Can you work these out from the model? Positions are in its coordinate system, mm. Give positions to 0.01 mm unless a question says otherwise; leave off trailing zeros. Order: outer loops, then holes, each group sorted by start corner. A loop starts at its lowest first (then second) coordinate and runs counter-clockwise, first axis right, second up. Notation, with made-up numbers: (43, 76) -> (64, 76) arc R36 cw to (64, 113) -> close; hole circle Ø2 at (67.5, 81). An arc over 180 degrees is marked (long way). Answer as a JSON object with one key per item and string values.
```python
from build123d import *

# Parameters (mm, degrees)
BOSS_EXTRUDE1_DEPTH                          = 2.5
CSK_FOR_M3_COUNTERSUNK_FLAT_HEAD_SCR_2_COUNT = 2
CSK_FOR_M3_COUNTERSUNK_FLAT_HEAD_SCR_2_PITCH = 33.1
CSK_FOR_M3_COUNTERSUNK_FLAT_HEAD_SCR_3_COUNT = 2
CSK_FOR_M3_COUNTERSUNK_FLAT_HEAD_SCR_3_PITCH = 73.026544956
CSK_FOR_M3_COUNTERSUNK_FLAT_HEAD_SCR_4_COUNT = 2
CSK_FOR_M3_COUNTERSUNK_FLAT_HEAD_SCR_4_PITCH = 146.05
CSK_FOR_M3_COUNTERSUNK_FLAT_HEAD_SCR_5_COUNT = 2
CSK_FOR_M3_COUNTERSUNK_FLAT_HEAD_SCR_5_PITCH = 149.753839684
CUT_EXTRUDE1_DEPTH                           = 86.383473485


with BuildPart() as part:
    # Sketch2 → Boss-Extrude1 (new body)
    with BuildSketch(Plane.XY):
        with BuildLine():
            Line((-75.2, -11.559818622), (75.2, -11.559818622))
            ThreePointArc((75.2, -11.559818622), (75.907106781, -11.266925403), (76.2, -10.559818622))
            Line((76.2, -10.559818622), (76.2, 37.440181378))
            ThreePointArc((76.2, 37.440181378), (75.907106781, 38.147288159), (75.2, 38.440181378))
            Line((75.2, 38.440181378), (-75.2, 38.440181378))
            ThreePointArc((-75.2, 38.440181378), (-75.907106781, 38.147288159), (-76.2, 37.440181378))
            Line((-76.2, 37.440181378), (-76.2, -10.559818622))
            ThreePointArc((-76.2, -10.559818622), (-75.907106781, -11.266925403), (-75.2, -11.559818622))
        make_face()
    extrude(amount=BOSS_EXTRUDE1_DEPTH)

    # Sketch5 → CSK for M3 Countersunk Flat Head Screw1 (revolve, cut)
    with BuildSketch(Plane(origin=(-73.025, 33.440181378, 2.5), x_dir=(0, -1, 0), z_dir=(1, 0, 0))):
        Polygon((0, 0), (0, 2.5), (1.7, 2.5), (1.7, 1.45), (3.15, 0), align=None)
    csk_for_m3_countersunk_flat_head_screw1 = revolve(axis=Axis((-73.025, 33.440181378, 8.85), (0, 0, -1)), mode=Mode.SUBTRACT)

    # CSK for M3 Countersunk Flat Head Scr 2: CSK for M3 Countersunk Flat Head Screw1 ×2
    with Locations(*[(0, -i * CSK_FOR_M3_COUNTERSUNK_FLAT_HEAD_SCR_2_PITCH, 0) for i in range(1, CSK_FOR_M3_COUNTERSUNK_FLAT_HEAD_SCR_2_COUNT)]):
        add(csk_for_m3_countersunk_flat_head_screw1, mode=Mode.SUBTRACT)

    # CSK for M3 Countersunk Flat Head Scr 3: CSK for M3 Countersunk Flat Head Screw1 ×2
    with Locations(*[Vector(0.9999788439186126, 0.006504745590340633, 0) * (i * CSK_FOR_M3_COUNTERSUNK_FLAT_HEAD_SCR_3_PITCH) for i in range(1, CSK_FOR_M3_COUNTERSUNK_FLAT_HEAD_SCR_3_COUNT)]):
        add(csk_for_m3_countersunk_flat_head_screw1, mode=Mode.SUBTRACT)

    # CSK for M3 Countersunk Flat Head Scr 4: CSK for M3 Countersunk Flat Head Screw1 ×2
    with Locations(*[(i * CSK_FOR_M3_COUNTERSUNK_FLAT_HEAD_SCR_4_PITCH, 0, 0) for i in range(1, CSK_FOR_M3_COUNTERSUNK_FLAT_HEAD_SCR_4_COUNT)]):
        add(csk_for_m3_countersunk_flat_head_screw1, mode=Mode.SUBTRACT)

    # CSK for M3 Countersunk Flat Head Scr 5: CSK for M3 Countersunk Flat Head Screw1 ×2
    with Locations(*[Vector(0.9752671471296755, -0.22102939109888511, 0) * (i * CSK_FOR_M3_COUNTERSUNK_FLAT_HEAD_SCR_5_PITCH) for i in range(1, CSK_FOR_M3_COUNTERSUNK_FLAT_HEAD_SCR_5_COUNT)]):
        add(csk_for_m3_countersunk_flat_head_screw1, mode=Mode.SUBTRACT)

    # Sketch6 → Cut-Extrude1 (cut, through all)
    with BuildSketch(Plane.XY.offset(2.5)):
        with BuildLine():
            ThreePointArc((-12.7, 7.935569815), (-16, 20.035569815), (-19.3, 7.935569815))
            Line((-19.3, 7.935569815), (-12.7, 7.935569815))
        make_face()
        with BuildLine():
            ThreePointArc((19.3, 7.935569815), (16, 20.035569815), (12.7, 7.935569815))
            Line((12.7, 7.935569815), (19.3, 7.935569815))
        make_face()
    extrude(amount=-CUT_EXTRUDE1_DEPTH, mode=Mode.SUBTRACT)


solid = part.part
```
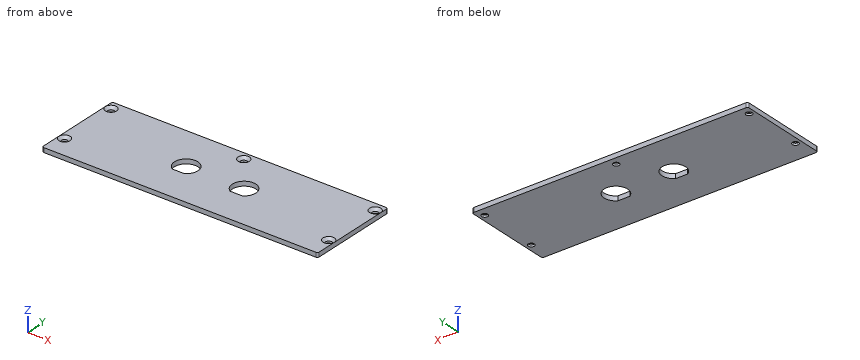
1. If we section it at D-D on x = 16: Please give me the cut outline in (y, z).
Worked answers:
{"outline": "(-11.56, 0) -> (7.94, 0) -> (7.94, 2.5) -> (-11.56, 2.5) -> close; (20.04, 0) -> (38.44, 0) -> (38.44, 2.5) -> (20.04, 2.5) -> close"}
2. If we section it at B-B on y = 13.5: Please give me the cut outline in (x, z).
Worked answers:
{"outline": "(-76.2, 0) -> (-22.5, 0) -> (-22.5, 2.5) -> (-76.2, 2.5) -> close; (-9.5, 0) -> (9.5, 0) -> (9.5, 2.5) -> (-9.5, 2.5) -> close; (22.5, 0) -> (76.2, 0) -> (76.2, 2.5) -> (22.5, 2.5) -> close"}
3. If we section it at C-C on z = 1.8: Please give me the cut outline in (x, y) (3 decimals).
Worked answers:
{"outline": "(-76.2, -10.56) arc R1 ccw to (-75.2, -11.56) -> (75.2, -11.56) arc R1 ccw to (76.2, -10.56) -> (76.2, 37.44) arc R1 ccw to (75.2, 38.44) -> (-75.2, 38.44) arc R1 ccw to (-76.2, 37.44) -> close; hole circle Ø4.9 at (-73.025, 0.34); hole circle Ø4.9 at (-73.025, 33.44); hole (-19.3, 7.936) -> (-12.7, 7.936) arc R6.5 ccw (long way) to start; hole circle Ø4.9 at (0, 33.915); hole (12.7, 7.936) -> (19.3, 7.936) arc R6.5 ccw (long way) to start; hole circle Ø4.9 at (73.025, 0.34); hole circle Ø4.9 at (73.025, 33.44)"}
4. If we section it at A-A on x = 0: Please give me the cut outline in (y, z).
Worked answers:
{"outline": "(-11.56, 0) -> (32.22, 0) -> (32.22, 1.05) -> (30.77, 2.5) -> (-11.56, 2.5) -> close; (35.62, 0) -> (38.44, 0) -> (38.44, 2.5) -> (37.07, 2.5) -> (35.62, 1.05) -> close"}
5. Will these pins go through, and if not, where does the flat tip stop? pin 1 Ø4.5 at (x, y) = (0, 33.92) entering from +Z; pin 2 Ø3 at (x, y) = (73.03, 0.34) entering from -Z.
Worked answers:
{"pin 1": "z = 1.6", "pin 2": "through"}
6. Please list where these lines run through material, in increasing order: L1, parallel to X at y = 13.5, z = 2.45; L2, parallel to X at y = 19, z = 1.9; L3, parallel to X at y = 35, z = 1.55.
Worked answers:
{"L1": "-76.2 to -22.5, -9.5 to 9.5, 22.5 to 76.2", "L2": "-76.2 to -19.52, -12.48 to 12.48, 19.52 to 76.2", "L3": "-76.2 to -74.58, -71.47 to -1.91, 1.91 to 71.47, 74.58 to 76.2"}
